Here's how the part is built. I have some questions about the finished solid (model axes, mm). Coordinates: 2 decimals unless noted, no trailing zeros. Loops run counter-clockwise (first coordinate to the right, second up) from the corner with the lowest first, then second, coordinate; pieces in that order, holes last. Notation, with made-up numbers: (-23.75, 67) -> (14.25, 67) arc R23 ccw to (14.25, 97) -> close; hole circle Ø1 at (-11, 73). An arc over 180 degrees is marked (long way). Answer as a JSON object with one key per item and string values. Group by question number.
Q1. I want a section at B-B on x = 347. Write out the boundary of the cut face in (y, z), then the cut area to 3 significant figures.
Q2. I need wall thicknesses on line 1 (X direction, y = -69.5, z = 0.45); line 2 (Y direction, x = 379, z = 1.25). Which ranges of each line are inside material? Lowest first, please.
Q3. I want a section at C-C on y = -141. Write out the boundary of the cut face in (x, z), then the cut area to 3 significant figures.
Q4. I want a section at A-A on z = 1.7. Write out the boundary of the cut face in (x, y), then the cut area to 3 significant figures.
Q5. I'm going to push flat-ended pins straight in: pin 1 (1 mm diameter, centred on y = -68, z = 1.5, fed in from +X); pin 2 (1.5 mm diameter, centred on x = 358, z = 1.5, fed in from -Y). Where does each tip first touch, or does it pass through?
```python
from build123d import *

# Parameters (mm, degrees)
F1_DEPTH = 3
F2_DEPTH = 25


with BuildPart() as f1:
    # F0 (on Top) → F1 (new body)
    with BuildSketch(Plane.XY):
        Polygon((201.401917, 185.517609), (-491.098083, 185.517609), (-491.098083, -251.482391), (194.901917, -251.482391), (194.901917, -51.482391), (464.901917, -51.482391), (464.901917, 185.517609), (328.401917, 185.517609), (264.901917, 185.517609), align=None)
        with BuildLine():
            ThreePointArc((264.901917, 184.017609), (264.401917, 184.517609), (264.901917, 185.017609))
            ThreePointArc((264.901917, 185.017609), (265.25547, 184.871162), (265.401917, 184.517609))
            ThreePointArc((265.401917, 184.517609), (265.25547, 184.164056), (264.901917, 184.017609))
        make_face(mode=Mode.SUBTRACT)
        with BuildLine():
            ThreePointArc((328.401917, 184.017609), (327.901917, 184.517609), (328.401917, 185.017609))
            ThreePointArc((328.401917, 185.017609), (328.75547, 184.871162), (328.901917, 184.517609))
            ThreePointArc((328.901917, 184.517609), (328.75547, 184.164056), (328.401917, 184.017609))
        make_face(mode=Mode.SUBTRACT)
    extrude(amount=F1_DEPTH)

    # F0 (on Top) → F2 (cut)
    with BuildSketch(Plane.XY):
        Polygon((201.401917, 185.517609), (-491.098083, 185.517609), (-491.098083, -251.482391), (194.901917, -251.482391), (194.901917, -51.482391), (464.901917, -51.482391), (464.901917, 185.517609), (328.401917, 185.517609), (264.901917, 185.517609), align=None)
        with BuildLine():
            ThreePointArc((264.901917, 184.017609), (264.401917, 184.517609), (264.901917, 185.017609))
            ThreePointArc((264.901917, 185.017609), (265.25547, 184.871162), (265.401917, 184.517609))
            ThreePointArc((265.401917, 184.517609), (265.25547, 184.164056), (264.901917, 184.017609))
        make_face(mode=Mode.SUBTRACT)
        with BuildLine():
            ThreePointArc((328.401917, 184.017609), (327.901917, 184.517609), (328.401917, 185.017609))
            ThreePointArc((328.401917, 185.017609), (328.75547, 184.871162), (328.901917, 184.517609))
            ThreePointArc((328.901917, 184.517609), (328.75547, 184.164056), (328.401917, 184.017609))
        make_face(mode=Mode.SUBTRACT)
    extrude(amount=-F2_DEPTH, mode=Mode.SUBTRACT)


solid = f1.part
```
Result set:
{
 "1": {"outline": "(-51.48, 0) -> (185.52, 0) -> (185.52, 3) -> (-51.48, 3) -> close", "area": "711 mm²"},
 "2": {"line 1": "x = -491.1 to 194.9", "line 2": "y = -51.48 to 185.52"},
 "3": {"outline": "(-491.1, 0) -> (194.9, 0) -> (194.9, 3) -> (-491.1, 3) -> close", "area": "2,060 mm²"},
 "4": {"outline": "(-491.1, -251.48) -> (194.9, -251.48) -> (194.9, -51.48) -> (464.9, -51.48) -> (464.9, 185.52) -> (-491.1, 185.52) -> close; hole (264.9, 184.02) arc R0.5 ccw to (265.4, 184.52) arc R0.5 ccw to (264.9, 185.02) arc R0.5 ccw to start; hole (328.4, 184.02) arc R0.5 ccw to (328.9, 184.52) arc R0.5 ccw to (328.4, 185.02) arc R0.5 ccw to start", "area": "364,000 mm²"},
 "5": {"pin 1": "stops at x = 194.9", "pin 2": "stops at y = -51.48"}
}
